Input: part model. Units: mm. Frame: model coordinates. Face numbers are marked on the shaded views. A direction names the side the tool comes from. Give positions to 0.01 mm unless a question says otherwise; leave off trailing zeros. Loops run counter-clockwise (first coordinate to the right, second up) from the corner with the lowest first, then second, coordinate; pieces in that order, holes last.
Autodesk Inventor part; units mm, degrees
ref_plane "YZ Plane" through (0, 0, 0) normal (1, 0, 0) x (0, 1, 0)
ref_plane "XZ Plane" through (0, 0, 0) normal (0, 1, 0) x (-1, 0, 0)
ref_plane "XY Plane" through (0, 0, 0) normal (0, 0, 1) x (1, 0, 0)
sketch "Sketch1" plane through (0, 0, 0) normal (0, 1, 0) x (-1, 0, 0)
  line L0 (0, 0) -> (76.2, 0)
  line L1 (76.2, 0) -> (76.2, -50.8)
  line L2 (76.2, -50.8) -> (0, -50.8)
  line L3 (0, -50.8) -> (0, 0)
  line L4 (76.2, -3.175) -> (0, -3.175)
  circle A0 centre (38.1, -25.4) radius 3.175
  dimension "d0" = 76.2
  dimension "d1" = 50.8
  dimension "d2" = 3.175
  dimension "d9" = 6.35
  dimension "d10" = 38.1
  dimension "d11" = 25.4
extrude "Extrusion1" add sketch "Sketch1" along normal blind 3.175 contours L4 L1 L2 L3
extrude "Extrusion2" add sketch "Sketch1" along normal blind 50.8 contours L0 L1 L4 L3
sketch "Sketch2" plane through (0, 50.8, 0) normal (0, 1, 0) x (1, 0, 0)
  line L0 (0, 50.8) -> (-76.2, 50.8)
  line L1 (0, 0) -> (-76.2, 0)
  line L2 (-76.2, 0) -> (-76.2, 50.8)
  line L3 (-76.2, 50.8) -> (0, 50.8)
  line L4 (0, 50.8) -> (0, 0)
  line L5 (-76.2, 50.8) -> (-76.2, 3.175)
  line L6 (0, 3.175) -> (0, 50.8)
  line L7 (-76.2, 3.175) -> (0, 3.175)
  circle A0 centre (-38.1, 25.4) radius 3.175
  circle A1 centre (-38.1, 25.4) radius 3.175
  dimension "d12" = 6.35
extrude "Extrusion3" add sketch "Sketch2" against normal blind 3.175 contours L4 L7 L2 L0
properties part number "Gear Shell"
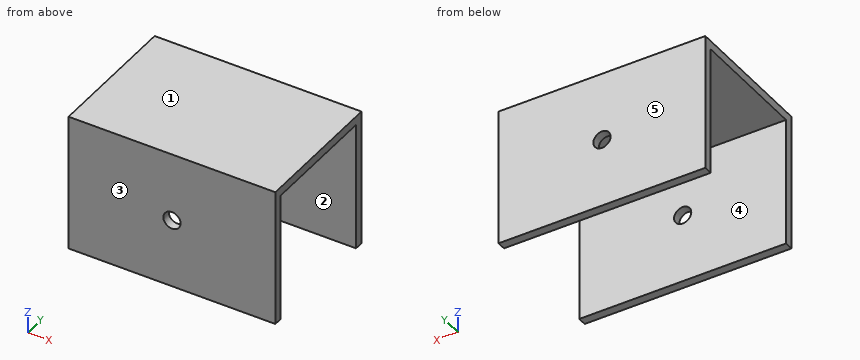
(1) Pin query (flat end, axial travel): pin 1 Ø14.5 at (x, z) = (-36.5, -17.5) entering from -Y; pin 2 Ø5 at (x, y) = (-51, 6) entering from -Z (3 decimals); pin 3 Ø1 at (y, z) = (45.5, -32) entering from +X. Return the tip coordinate at first contact, or that it passes through.
Values follow:
pin 1: stops at y = 0
pin 2: stops at z = -3.175
pin 3: passes through
(2) Cut plane C-C (z = -47). Return the cut outline in (x, y) (3 decimals).
Values follow:
outline: (-76.2, 0) - (0, 0) - (0, 3.175) - (-76.2, 3.175) - close; (-76.2, 47.625) - (0, 47.625) - (0, 50.8) - (-76.2, 50.8) - close
(3) Reachability of the marked faces 4 and 5 from +Z, -Z, +X, -X, +Y, -Y: full face, straight path, thin tool, end or side. Return the list, or none.
Values follow:
face 4: -Z, +X, -X
face 5: +Z, -Z, +X, -X, +Y
(4) Ray query, probe 1 along X at (y, z) = (49.6, -25.4) (3 decimals); probe 2 along Y at (x, z) = (-41, -15.5) (3 decimals); probe 3 along Z at (x, y) = (-38.1, 49.45) (3 decimals). Return the intervals inside material, ascending.
Values follow:
probe 1: x = -76.2 to -41.275, -34.925 to 0
probe 2: y = 0 to 3.175, 47.625 to 50.8
probe 3: z = -50.8 to -28.575, -22.225 to 0
(5) Cut plane A-A (x = -38.1). Return the cut outline in (y, z) (3 decimals), and give its area (3 significant figures).
Values follow:
outline: (0, -50.8) - (3.175, -50.8) - (3.175, -28.575) - (0, -28.575) - close; (0, -22.225) - (3.175, -22.225) - (3.175, -3.175) - (47.625, -3.175) - (47.625, -22.225) - (50.8, -22.225) - (50.8, 0) - (0, 0) - close; (47.625, -50.8) - (50.8, -50.8) - (50.8, -28.575) - (47.625, -28.575) - close
area: 423 mm2
(6) Cut plane D-D (x = -17). Return the cut outline in (y, z) (3 decimals).
Values follow:
outline: (0, -50.8) - (3.175, -50.8) - (3.175, -3.175) - (47.625, -3.175) - (47.625, -50.8) - (50.8, -50.8) - (50.8, 0) - (0, 0) - close
(7) Mould query, pull axis Y, two halves, no side actions, for the marked faces 1, 2 and 3. Classes: +Y half, -Y half, draft (parallel to the pull), parting line (faces both ways), or undercut.
Values follow:
face 1: draft
face 2: undercut
face 3: -Y half
(8) Cut plane B-B (z = -25.4). Return the cut outline in (x, y) (3 decimals), and give its area (3 significant figures).
Values follow:
outline: (-76.2, 0) - (-41.275, 0) - (-41.275, 3.175) - (-76.2, 3.175) - close; (-76.2, 47.625) - (-41.275, 47.625) - (-41.275, 50.8) - (-76.2, 50.8) - close; (-34.925, 0) - (0, 0) - (0, 3.175) - (-34.925, 3.175) - close; (-34.925, 47.625) - (0, 47.625) - (0, 50.8) - (-34.925, 50.8) - close
area: 444 mm2
